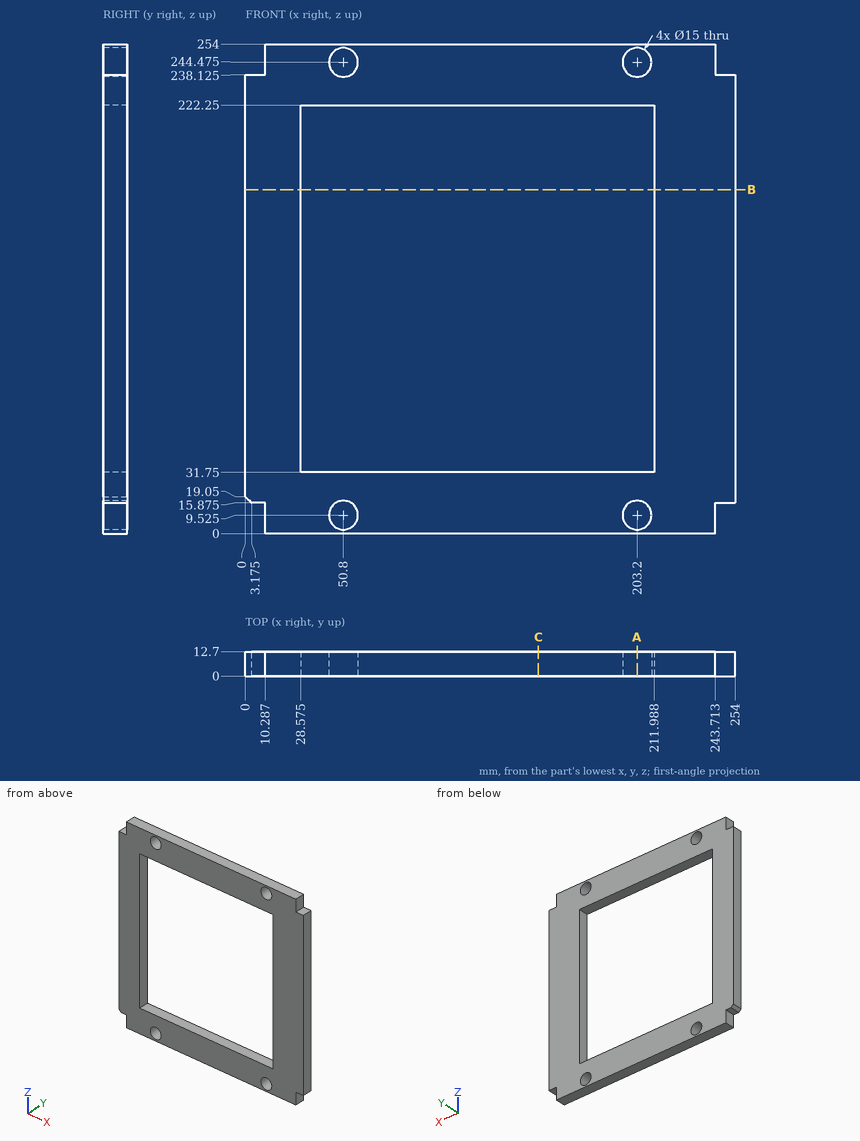
Print and shaded views of the part. All mm, measured from the part's lowest x, y and z. Give positions to 0.01 mm unless a question says otherwise; leave off trailing zeros. Order: outer loops, then holes, each group sorted by start corner. A loop starts at its lowest first (then second) coordinate and runs counter-clockwise, first axis right, second up. Notation, with made-up numbers: (61.25, 72) - (103.25, 72) arc R16 ccw to (103.25, 101) - close; hole circle Ø5 at (76.5, 89.5). An arc over 180 degrees is marked (long way). One line per item, written item: value.
Item 1: Slice it at A-A (x = 203.2). Give the number of separate pieces and of enclosed holes in the cut face.
Response values:
separate pieces: 4
enclosed holes: 0
Item 2: Slice it at C-C (x = 152). List the corners of the cut face in (y, z).
Response values:
outline: (0, 0) - (12.7, 0) - (12.7, 31.75) - (0, 31.75) - close; (0, 222.25) - (12.7, 222.25) - (12.7, 254) - (0, 254) - close
Item 3: Pin check, flat tips, straight feed: pin 1 Ø4 at (y, z) = (5.5, 4) entering from +X; pin 2 Ø3 at (x, y) = (3, 6.5) entering from +Z (3 decimals); pin 3 Ø2 at (x, y) = (7.5, 6) entering from -Z (3 decimals). Stop position of each tip, or through.
Response values:
pin 1: x = 243.71
pin 2: z = 238.125
pin 3: z = 15.875
Item 4: Wall check: line 1 (X direction, y = 7.5, z = 78) (1 decimal); line 2 (Z direction, x = 79, y = 0.5); line 3 (Z direction, x = 209, y = 6). Give the ranges that are in metal, low to high.
Response values:
line 1: 0 to 28.6, 212 to 254
line 2: 0 to 31.75, 222.25 to 254
line 3: 0 to 4.77, 14.28 to 31.75, 222.25 to 239.72, 249.23 to 254
Item 5: Slice it at B-B (z = 178.5). List the corners of the cut face in (x, y) (1 decimal).
Response values:
outline: (0, 0) - (28.6, 0) - (28.6, 12.7) - (0, 12.7) - close; (212, 0) - (254, 0) - (254, 12.7) - (212, 12.7) - close
